```python
from build123d import *

# Parameters (mm, degrees)
SKETCH1_R           = 4
BOSS_EXTRUDE1_DEPTH = 3
SKETCH2_R           = 6.5
BOSS_EXTRUDE2_DEPTH = 52
SKETCH3_R           = 3.5
CUT_EXTRUDE1_DEPTH  = 90.364422451
CHAMFER1_SIZE       = 1


with BuildPart() as part:
    # Sketch1 → Boss-Extrude1 (new body)
    with BuildSketch(Plane.XY):
        with BuildLine():
            Line((27.5, 29.5), (51, 29.5))
            Line((51, 29.5), (51, 10))
            ThreePointArc((51, 10), (48.071067812, 2.928932188), (41, 0))
            Line((41, 0), (-41, 0))
            ThreePointArc((-41, 0), (-48.071067812, 2.928932188), (-51, 10))
            Line((-51, 10), (-51, 29.5))
            Line((-51, 29.5), (-27.5, 29.5))
            ThreePointArc((-27.5, 29.5), (-26.439339828, 29.939339828), (-26, 31))
            Line((-26, 31), (-26, 37.5))
            Line((-26, 37.5), (26, 37.5))
            Line((26, 37.5), (26, 31))
            ThreePointArc((26, 31), (26.439339828, 29.939339828), (27.5, 29.5))
        make_face()
        with Locations((-38, 19)):
            Circle(SKETCH1_R, mode=Mode.SUBTRACT)
        with Locations((38, 19)):
            Circle(SKETCH1_R, mode=Mode.SUBTRACT)
        with Locations((-12.5, 10)):
            Circle(SKETCH1_R, mode=Mode.SUBTRACT)
        with Locations((12.5, 10)):
            Circle(SKETCH1_R, mode=Mode.SUBTRACT)
    extrude(amount=BOSS_EXTRUDE1_DEPTH)

    # Sketch2 → Boss-Extrude2 (add)
    with BuildSketch(Plane.ZY.offset(26)):
        with Locations((4.5, 37.5)):
            Circle(SKETCH2_R)
    extrude(amount=-BOSS_EXTRUDE2_DEPTH)

    # Sketch3 → Cut-Extrude1 (cut, through all)
    with BuildSketch(Plane.ZY.offset(26)):
        with Locations((4.5, 37.5)):
            Circle(SKETCH3_R)
    extrude(amount=-CUT_EXTRUDE1_DEPTH, mode=Mode.SUBTRACT)

    # Chamfer1
    chamfer1_edges = [part.edges().sort_by_distance(p)[0] for p in [
        (-42, 19, 3),
        (34, 19, 3),
        (-16.5, 10, 3),
        (8.5, 10, 3),
    ]]
    chamfer(chamfer1_edges, length=CHAMFER1_SIZE)


solid = part.part
```
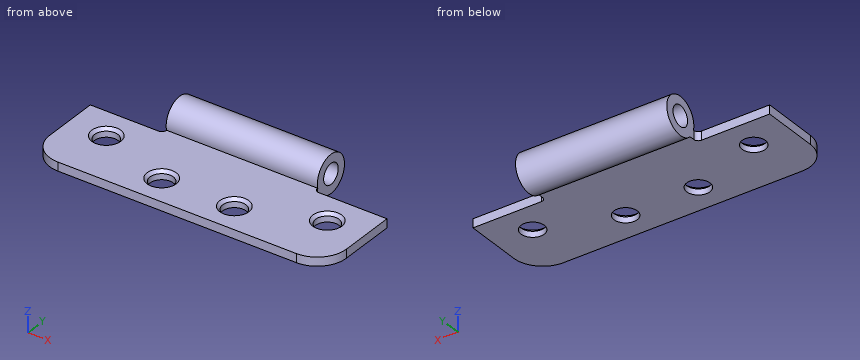
The model under review builds one solid part; all positions refer to its coordinate system, in mm. Give positions to 0.01 mm unless a question says otherwise; leave off trailing zeros. Write each loop counter-clockwise with the first axis right and the second up, starting at its lowest first coordinate (ties: lowest second). Pieces come first, ordered by that corner, then holes. Notation, with made-up numbers: M 30,23 L 35,23 A23 ccw 35,60 Z; hole C 38.25,67 d3. An arc over 180 degrees is marked long. Write item = value, one per line. Start each with the question number.
Q1. We need section D-D (y = 37.5). State the section outline as (x, z) points, plus the area to 3 significant figures.
Q2. We need section A-A (x = -12.5). State the section outline as (y, z) points.
Q3. We need section B-B (z = 4.5). State the section outline as (x, y) points, plus the area to 3 significant figures.
Q4. Clearance check with flat-ended pins moving along their axes: pin 1 (1.5 mm diameter, centred on x = -38, z = 1, fed in from +Y); pin 2 (1.5 mm diameter, centred on x = -28.5, y = 5.5, fed in from -Z); pin 3 (6 mm diameter, centred on x = 13, z = -0.5, fed in from +Y). State where each tip first meets the part, or that it passes through.
Q5. We need section C-C (x = 38). State the section outline as (y, z) points.
Q6. For line 1 (Y direction, x = 12.5, z = 1.4); line 2 (Z direction, x = 9.5, y = 27); line 3 (X direction, y = 18, z = 2), list the stretches that pass through material, from the lowest coordinate up.
Result set:
q1.outline = M -26,-2 L 26,-2 L 26,1 L -26,1 Z; M -26,8 L 26,8 L 26,11 L -26,11 Z
q1.area = 312 mm2
q2.outline = M 0,0 L 6,0 L 6,2 L 5,3 L 0,3 Z; M 14,0 L 32.81,0 A6.5 ccw long 31.18,3 L 15,3 L 14,2 Z; hole C 37.5,4.5 d7
q3.outline = M -26,31 L 26,31 L 26,34 L -26,34 Z; M -26,41 L 26,41 L 26,44 L -26,44 Z
q3.area = 312 mm2
q4.pin_1 = 29.5
q4.pin_2 = 0
q4.pin_3 = 43.68
q5.outline = M 0,0 L 15,0 L 15,2 L 14,3 L 0,3 Z; M 23,0 L 29.5,0 L 29.5,3 L 24,3 L 23,2 Z
q6.line_1 = 0 to 6, 14 to 35.88, 39.12 to 43.21
q6.line_2 = 0 to 3
q6.line_3 = -51 to -41.87, -34.13 to 34.13, 41.87 to 51
